Drawing for the job (mm, zero at the part's lowest x, y, z). A direction names the side the tool comes from. Coordinates: 2 decimals unless noted, no trailing zeros. Loops run counter-clockwise (first coordinate to the right, second up) from the corner with the lowest first, then second, coordinate; pieces in that order, holes last. Notation, with made-up numbers: (-23.75, 18) -> (-11.75, 18) arc R21 ccw to (-11.75, 52) -> close; hole circle Ø11 at (-32, -19). An arc over 180 degrees is marked (long way). Write item = value, one per line. Start each with the question number.
(1) Band-saw the part on C-C (y = 39.5). Write the cut outline in (x, z) (1 decimal).
(2) Drill centre lines: line 1 (Y direction, x = 85.5, z = 14.75); line 2 (Z direction, x = 44.5, y = 37); line 3 (X direction, y = 48, z = 11.75). Where is each one in solid material? Low to high. Write a range as from..to.
(3) Band-saw the part on A-A (x = 105). Write the cut outline in (y, z), and give its area (3 significant figures).
(4) Band-saw the part on D-D (x = 69.5). Write the cut outline in (y, z).
(5) Flat gauge pins, fed straight in: P1, Ø8, axis at y = 78, z = 11.5, coming from the +X side; P2, Ø12, axis at y = 57.5, z = 25.5, coming from the -X side; P3, Ø5, axis at x = 90, z = 13.5, coming from the +Y side. Where does each tip first touch, or does it go through?
(6) Band-saw the part on B-B (z = 2). Write the cut outline in (x, y), and give its area (4 significant figures).
(7) Tool access for the marked faces 1, 2, 3, 4 and 5: list every direction of +Z, -Z, +X, -X, +Y, -Y with a clear straight run to the whole face (end or side of a thin tool).
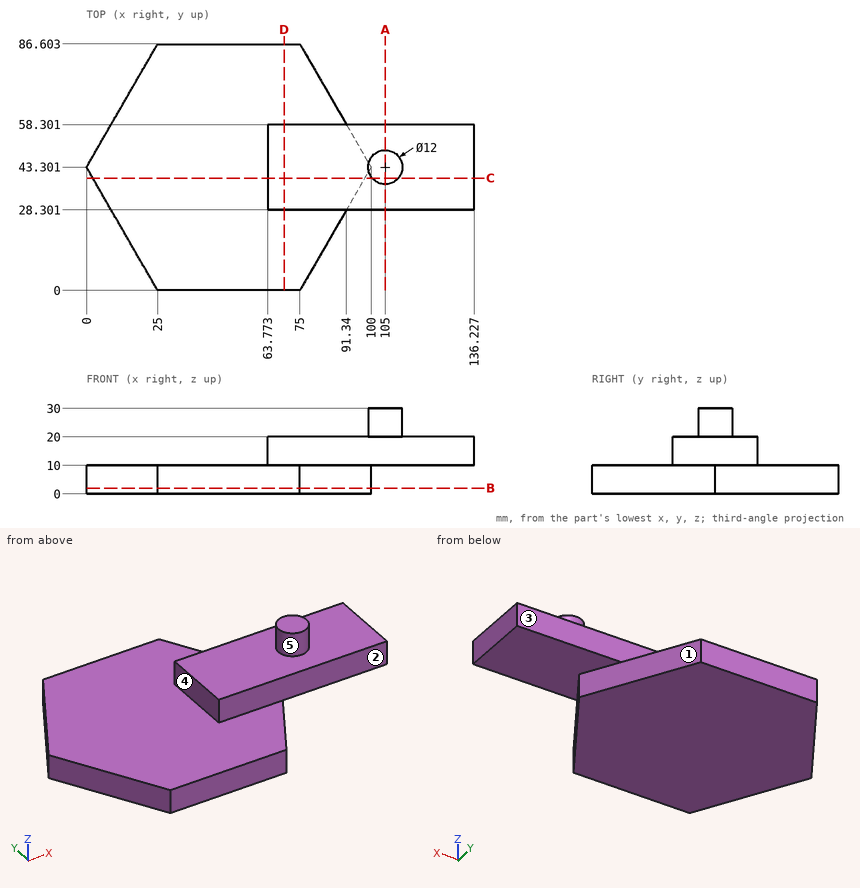
Findings below:
q1.outline = (2.2, 0) -> (97.8, 0) -> (97.8, 10) -> (136.2, 10) -> (136.2, 20) -> (109.6, 20) -> (109.6, 30) -> (100.4, 30) -> (100.4, 20) -> (63.8, 20) -> (63.8, 10) -> (2.2, 10) -> close
q2.line_1 = 28.3..58.3
q2.line_2 = 0..10
q2.line_3 = 63.77..136.23
q3.outline = (28.3, 10) -> (58.3, 10) -> (58.3, 20) -> (49.3, 20) -> (49.3, 30) -> (37.3, 30) -> (37.3, 20) -> (28.3, 20) -> close
q3.area = 420 mm²
q4.outline = (0, 0) -> (86.6, 0) -> (86.6, 10) -> (58.3, 10) -> (58.3, 20) -> (28.3, 20) -> (28.3, 10) -> (0, 10) -> close
q5.P1 = 82.11
q5.P2 = 63.77
q5.P3 = 58.3
q6.outline = (0, 43.3) -> (25, 0) -> (75, 0) -> (100, 43.3) -> (75, 86.6) -> (25, 86.6) -> close
q6.area = 6,495 mm²
q7.face_1 = -Z, +X, +Y
q7.face_2 = +Z, +X, -X, -Y
q7.face_3 = +Z, +X, -X, +Y
q7.face_4 = +Z, -X, +Y, -Y
q7.face_5 = +Z
